```python
from build123d import *

# Parameters (mm, degrees)
F0_R      = 7.5
F1_DEPTH  = 30
F2_R      = 4.25
F3_DEPTH  = 20
F4_R      = 4.25
F5_DEPTH  = 3
F7_R      = 7.5
F8_DEPTH  = 10
F10_DEPTH = 3


# Not quite as in the source:
# - a feature names something its author has since deleted; it is built from what else it names


with BuildPart() as f1:
    # F0 (on Top) → F1 (new body)
    with BuildSketch(Plane.XY):
        Circle(F0_R)
    extrude(amount=F1_DEPTH)

    # F2 (on face) → F3 (cut)
    with BuildSketch(Plane(origin=(0, 0, 0), x_dir=(1, 0, 0), z_dir=(0, 0, -1))):
        Circle(F2_R)
    extrude(amount=-F3_DEPTH, mode=Mode.SUBTRACT)

    # F4 (on face) → F5 (cut)
    with BuildSketch(Plane(origin=(0, 0, 0), x_dir=(1, 0, 0), z_dir=(0, 0, -1))):
        Polygon((5.8, -3.3486315613), (5.8, 3.3486315613), (0, 6.6972631226), (-5.8, 3.3486315613), (-5.8, -3.3486315613), (0, -6.6972631226), align=None)
        Circle(F4_R, mode=Mode.SUBTRACT)
    extrude(amount=-F5_DEPTH, mode=Mode.SUBTRACT)

    # F7 (on face) → F8 (cut)
    with BuildSketch(Plane.XY.offset(30)):
        Circle(F7_R)
        Polygon((0, 7.0436732841), (6.1, 3.5218366421), (6.1, -3.5218366421), (0, -7.0436732841), (-6.1, -3.5218366421), (-6.1, 3.5218366421), align=None, mode=Mode.SUBTRACT)
    extrude(amount=-F8_DEPTH, mode=Mode.SUBTRACT)

    # F9 (on face) → F10 (cut, through all)
    with BuildSketch(Plane(origin=(0, 0, 0), x_dir=(1, 0, 0), z_dir=(0, 0, -1))):
        with BuildLine():
            Line((4.1120525285, 6.2722423425), (5.8, 3.3486315613))
            Line((5.8, 3.3486315613), (5.8, -3.3486315613))
            Line((5.8, -3.3486315613), (0, -6.6972631226))
            Line((0, -6.6972631226), (-3.3758949431, -6.6972631226))
            ThreePointArc((-3.3758949431, -6.6972631226), (3.9326065101, -6.3862826462), (7.5, 0))
            ThreePointArc((7.5, 0), (6.5988784639, 3.5643797523), (4.1120525285, 6.2722423425))
        make_face()
    extrude(amount=-F10_DEPTH, mode=Mode.SUBTRACT)


solid = f1.part
```
Verification items for the finished model (mm, model axes). A direction names the side the tool comes from. Coordinates: 2 decimals unless noted, no trailing zeros. Loops run counter-clockwise (first coordinate to the right, second up) from the corner with the lowest first, then second, coordinate; pieces in that order, holes last. Notation, with made-up numbers: (-14, -3) -> (4, -3) arc R28 ccw to (4, 18) -> close; hole circle Ø4 at (8.25, 76.25). An arc over 180 degrees is marked (long way). Answer in a Markdown table with one row per item. Add a question column.
1. Access from +Z, -Z, +X, -X, +Y, -Y to the whole of each face (thin tool, end or side, straight path). Record for faces 5 (the face through (2.94, -5, 1.48)), 6 (the face through (-3.007, -5.307, 25.07)), 7 (the face through (2.285, -3.584, 11.381)).
2. Material ranges on probe 1 along Y at (x, z) = (0, 13.75); probe 2 along Z at (x, y) = (4, 4.25), recorded low to high. Write a range as [from, to].
3. Section check B-B, the plane z = 7. Enter the section's corners in (x, y), then the cut area to 3 significant figures.
4. Section check C-C, the plane x = 3.75. Enter the section's corners in (y, z).
5. Draft check along Y on faces 1 (the face through (-6, -2, 0)), 2 (the face through (4.944, -4.831, 1.479)), 3 (the face through (4, -3, 3)), 4 (the face through (-3.09, 5.26, 25.07)). Enter one of: +Y half, -Y half, draft (parallel to the pull), parting line (faces both ways), or undercut.
6. Depth check by flat-ended pin: P1, Ø4, axis at x = -1, y = 1.5, coming from the -Z side; P2, Ø1, axis at x = -4.5, y = 0.5, coming from the -Z side; P3, Ø4, axis at y = -3, z = 15, coming from the -X side. Enter the tip coordinate at first touch or a pass-through.
7. Section check A-A, the plane y = 0. Enter the section's corners in (x, z).
8. Section check D-D, the plane z = 21.25. Enter the section's corners in (x, y).
Derived:
| question | item | result |
|---|---|---|
| 1 | face 5 | -Z, +Y |
| 1 | face 6 | +Z, -X, -Y |
| 1 | face 7 | -Z |
| 2 | probe 1 | y = [-7.5, -4.25], [4.25, 7.5] |
| 2 | probe 2 | z = [3, 30] |
| 3 | outline | circle Ø15 at (0, 0); hole circle Ø8.5 at (0, 0) |
| 3 | area | 120 mm² |
| 4 | outline | (-6.5, 0) -> (-4.53, 0) -> (-4.53, 3) -> (-2, 3) -> (-2, 20) -> (2, 20) -> (2, 3) -> (6.5, 3) -> (6.5, 20) -> (4.88, 20) -> (4.88, 30) -> (-4.88, 30) -> (-4.88, 20) -> (-6.5, 20) -> close |
| 5 | face 1 | draft |
| 5 | face 2 | -Y half |
| 5 | face 3 | undercut |
| 5 | face 4 | +Y half |
| 6 | P1 | stops at z = 20 |
| 6 | P2 | stops at z = 3 |
| 6 | P3 | stops at x = -7.43 |
| 7 | outline | (-7.5, 0) -> (-5.8, 0) -> (-5.8, 3) -> (-4.25, 3) -> (-4.25, 20) -> (4.25, 20) -> (4.25, 3) -> (7.5, 3) -> (7.5, 20) -> (6.1, 20) -> (6.1, 30) -> (-6.1, 30) -> (-6.1, 20) -> (-7.5, 20) -> close |
| 8 | outline | (-6.1, -3.52) -> (0, -7.04) -> (6.1, -3.52) -> (6.1, 3.52) -> (0, 7.04) -> (-6.1, 3.52) -> close |
